```python
from build123d import *

# Parameters (mm, degrees)
CYLINDER098_R     = 6
CYLINDER098_DEPTH = 15
CYLINDER096_R     = 4.1
CYLINDER096_DEPTH = 15
BOX053_W          = 11.2
BOX053_H          = 8.5
BOX053_DEPTH      = 15
CYLINDER097_R     = 5.6
CYLINDER097_DEPTH = 15


with BuildPart() as zylinder089:
    # Cylinder098 → Cylinder098 (new body)
    with BuildSketch(Plane(origin=(0, -6, 0), x_dir=(1, 0, 0), z_dir=(0, 0, 1))):
        Circle(CYLINDER098_R)
    extrude(amount=CYLINDER098_DEPTH)


with BuildPart() as zylinder087:
    # Cylinder096 → Cylinder096 (new body)
    with BuildSketch(Plane.XY):
        Circle(CYLINDER096_R)
    extrude(amount=CYLINDER096_DEPTH)


with BuildPart() as obj1:
    # Box053 → Box053 (new body)
    with BuildSketch(Plane(origin=(-5.6, 0, 0), x_dir=(1, 0, 0), z_dir=(0, 0, 1))):
        with Locations((5.6, 4.25)):
            Rectangle(BOX053_W, BOX053_H)
    extrude(amount=BOX053_DEPTH)


with BuildPart() as cut011004014002011:
    # Cylinder097 → Cylinder097 (new body)
    with BuildSketch(Plane.XY):
        Circle(CYLINDER097_R)
    extrude(amount=CYLINDER097_DEPTH)

    # Fusion026038: union obj1
    add(obj1.part)

    # Cut011004014002010: cut Zylinder087
    add(zylinder087.part, mode=Mode.SUBTRACT)

    # Cut011004014002011: cut Zylinder089
    add(zylinder089.part, mode=Mode.SUBTRACT)


solid = cut011004014002011.part
```
Could you check a few things on this model? Use its own coordinates, in mm. A direction names the side the tool comes from. Coordinates: 2 decimals unless noted, no trailing zeros. Loops run counter-clockwise (first coordinate to the right, second up) from the corner with the lowest first, then second, coordinate; pieces in that order, holes last.
1) Please list where these lines run through material, in increasing order: line 1 along X through (y, z) = (0, 8); line 2 along Y through (x, z) = (0, 4.5); line 3 along X through (y, z) = (-1, 4).
Reported:
line 1: x = -5.6 to -4.1, 4.1 to 5.6
line 2: y = 4.1 to 8.5
line 3: x = -5.51 to -3.98, 3.98 to 5.51
2) Imagine slicing it at B-B (y = 1.5). List the corners of the cut face in (x, z) for me, and give its area (3 significant figures).
Reported:
outline: (-5.6, 0) - (-3.82, 0) - (-3.82, 15) - (-5.6, 15) - close; (3.82, 0) - (5.6, 0) - (5.6, 15) - (3.82, 15) - close
area: 53.5 mm2
3) Which directions (+Z, -Z, +X, -X, +Y, -Y) give clear straight access to the entire face, cutting with the end or side of a thin tool? Please do faces 5 (the face through (-0.1, 4.3, 0)), 6 (the face through (4.452, -1.978, 7.395)).
Reported:
face 5: -Z, +X, -X, +Y, -Y
face 6: +Z, -Z, -Y
4) Imagine slicing it at D-D (y = 3.25). List the corners of the cut face in (x, z) for me.
Reported:
outline: (-5.6, 0) - (-2.5, 0) - (-2.5, 15) - (-5.6, 15) - close; (2.5, 0) - (5.6, 0) - (5.6, 15) - (2.5, 15) - close
5) Imagine slicing it at A-A (z = 9.25). List the corners of the cut face in (x, y) for me.
Reported:
outline: (-5.6, 0) arc R5.6 ccw to (-4.95, -2.61) arc R6 cw to (-3.85, -1.4) arc R4.1 cw (long way) to (3.85, -1.4) arc R6 cw to (4.95, -2.61) arc R5.6 ccw to (5.6, 0) - (5.6, 8.5) - (-5.6, 8.5) - close
6) Imagine slicing it at C-C (x = 0). List the corners of the cut face in (y, z) for me, and give its area (3 significant figures).
Reported:
outline: (4.1, 0) - (8.5, 0) - (8.5, 15) - (4.1, 15) - close
area: 66.0 mm2
7) Thinking about a two-plate mould opening in Y: for faces 1 (the face through (-4.437, -1.961, 7.395)), 2 (the face through (0.1, 4.1, 7.4)), 3 (the face through (0, 8.5, 7)), 4 (the face through (-0.1, 4.3, 15)), which applies, released by +Y, released by -Y, zero draft, split by the parting line, or undercut?
Reported:
face 1: released by -Y
face 2: undercut
face 3: released by +Y
face 4: zero draft
